Input: part model. Units: mm. Frame: model coordinates. A direction names the side the tool comes from. Coordinates: 2 decimals unless noted, no trailing zeros. Loops run counter-clockwise (first coordinate to the right, second up) from the corner with the lowest first, then second, coordinate; pieces in that order, holes last.
```python
from build123d import *

# Parameters (mm, degrees)
F0_W     = 400
F0_H     = 300
F1_DEPTH = 25
F2_T     = -19
F3_SIZE  = 5
F5_R     = 41.152145
F4_DEPTH = 138.924479


with BuildPart() as f1:
    # F0 (on Top) → F1 (new body)
    with BuildSketch(Plane.XY):
        Rectangle(F0_W, F0_H)
    extrude(amount=F1_DEPTH)

    # F2
    f2_openings = [f1.faces().sort_by_distance(p)[0] for p in [
        (0, 0, 25),
    ]]
    offset(amount=F2_T, openings=f2_openings)

    # F3
    f3_edges = [f1.edges().sort_by_distance(p)[0] for p in [
        (-200, 0, 25),
        (0, 150, 25),
        (200, 0, 25),
        (0, -150, 25),
    ]]
    chamfer(f3_edges, length=F3_SIZE)

    # F5 (on face) → F4 (join)
    with BuildSketch(Plane.XY.offset(19)):
        with Locations((0, -63.907109)):
            Circle(F5_R)
    extrude(amount=F4_DEPTH)


solid = f1.part
```
Item 1: Contact query for flat-ended pins moving along their axis: P1, Ø5, axis at x = 83.5, y = 26.5, coming from the +Z side; P2, Ø2, axis at y = -52.5, z = 126.5, coming from the -X side; P3, Ø1, axis at x = 8, z = 120.5, coming from the -Y side. Output: stop coordinate, or through.
Result:
P1: stops at z = 19
P2: stops at x = -39.81
P3: stops at y = -104.37
Item 2: Section query C-C (x = 77.5). Output: boundary loops of the cut face in (y, z).
Result:
outline: (-150, 0) - (150, 0) - (150, 20) - (145, 25) - (131, 25) - (131, 19) - (-131, 19) - (-131, 25) - (-145, 25) - (-150, 20) - close
Item 3: Reachability of faces 1 (the face through (-3, 2, 0)), 2 (the face through (18.989, -100.416, 87.49)) from +Z, -Z, +X, -X, +Y, -Y: full face, straight path, thin tool, end or side. Return the list, or none.
Result:
face 1: -Z, +X, -X, +Y, -Y
face 2: +Z
Item 4: Section query A-A (x = 0). Output: boundary loops of the cut face in (y, z), then the cut area to 3 significant figures.
Result:
outline: (-150, 0) - (150, 0) - (150, 20) - (145, 25) - (131, 25) - (131, 19) - (-22.75, 19) - (-22.75, 157.92) - (-105.06, 157.92) - (-105.06, 19) - (-131, 19) - (-131, 25) - (-145, 25) - (-150, 20) - close
area: 17,300 mm2
Item 5: Mould query, pull axis X, two halves, no side actions, for faces 3 (the face through (-3, 150, 10)), 4 (the face through (-3, 2, 19)), 5 (the face through (200, -2, 10)), 6 (the face through (-200, -2, 10)). Classes: +X half, -X half, draft (parallel to the pull), parting line (faces both ways), or undercut.
Result:
face 3: draft
face 4: undercut
face 5: +X half
face 6: -X half
Item 6: Line query: L1, parallel to Z at x = 138.5, y = 44.5; L2, parallel to Z at x = 182, y = -46.5; L3, parallel to Y at x = 10, z = 85. Output: solid intervals per line, ascending.
Result:
L1: z = 0 to 19
L2: z = 0 to 25
L3: y = -103.83 to -23.99
Item 7: Section query B-B (y = 24). Output: boundary loops of the cut face in (x, z).
Result:
outline: (-200, 0) - (200, 0) - (200, 20) - (195, 25) - (181, 25) - (181, 19) - (-181, 19) - (-181, 25) - (-195, 25) - (-200, 20) - close
Item 8: Section query D-D (y = -48.5). Output: boundary loops of the cut face in (x, z), then the cut area to 3 significant figures.
Result:
outline: (-200, 0) - (200, 0) - (200, 20) - (195, 25) - (181, 25) - (181, 19) - (38.16, 19) - (38.16, 157.92) - (-38.16, 157.92) - (-38.16, 19) - (-181, 19) - (-181, 25) - (-195, 25) - (-200, 20) - close
area: 18,400 mm2
